Verification items for the finished model (mm, model axes). Face numbers are marked on the shaded views. A direction names the side the tool comes from. Round coordinates to 2 decimals unless told otherwise and drop trailing zeros. Write each loop counter-clockwise with the first axis right and the second up, starting at its lowest first coordinate (ties: lowest second). Pieces come first, ordered by that corner, then holes. Notation, with made-up numbers: (68.25, -22) - (94.25, -22) arc R12 ccw to (94.25, -3) - close; hole circle Ø8 at (72, 68). An arc over 180 degrees is marked (long way). Answer as a JSON object with one key per item and string values.
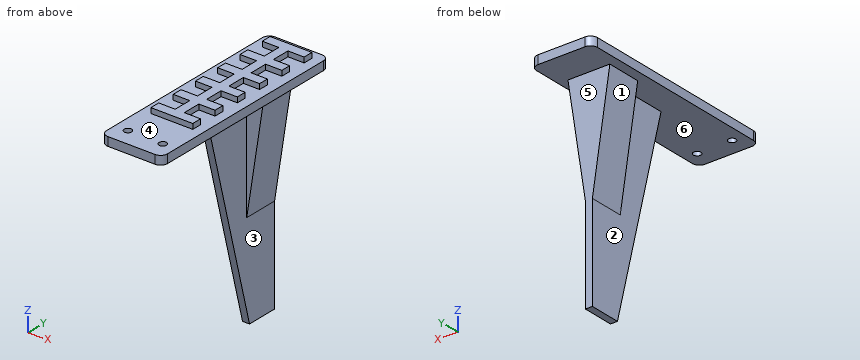
```python
from build123d import *

# Parameters (mm, degrees)
SKETCH1_W           = 15
SKETCH1_H           = 100
SKETCH1_W_2         = 35
SKETCH1_H_2         = 20
BOSS_EXTRUDE1_DEPTH = 5
SKETCH3_R           = 2.15
CUT_EXTRUDE1_DEPTH  = 6
BOSS_EXTRUDE3_DEPTH = 5
BOSS_EXTRUDE4_DEPTH = 2
BOSS_EXTRUDE5_DEPTH = 5
BOSS_EXTRUDE6_DEPTH = 20
FILLET3_R           = 4
BOSS_EXTRUDE7_DEPTH = 3


with BuildPart() as part:
    # Sketch1 → Boss-Extrude1 (new body)
    with BuildSketch(Plane.XY):
        with Locations((17.5, 50)):
            Rectangle(SKETCH1_W, SKETCH1_H)
        with Locations((17.5, -10)):
            Rectangle(SKETCH1_W_2, SKETCH1_H_2)
    extrude(amount=BOSS_EXTRUDE1_DEPTH)

    # Sketch3 → Cut-Extrude1 (cut, through all)
    with BuildSketch(Plane(origin=(0, 0, 0), x_dir=(-1, 0, 0), z_dir=(0, 0, -1))):
        with Locations((-27.5, -10)):
            Circle(SKETCH3_R)
        with Locations((-7.5, -10)):
            Circle(SKETCH3_R)
    extrude(amount=-CUT_EXTRUDE1_DEPTH, mode=Mode.SUBTRACT)

    # Sketch4 → Boss-Extrude3 (add)
    with BuildSketch(Plane(origin=(0, 0, 0), x_dir=(-1, 0, 0), z_dir=(0, 0, -1))):
        Polygon((-35, 0), (-25, 0), (-25, 62), align=None)
        Polygon((-10, 62), (0, 0), (-10, 0), align=None)
    extrude(amount=-BOSS_EXTRUDE3_DEPTH)

    # Sketch5 → Boss-Extrude4 (add, symmetric)
    with BuildSketch(Plane.ZY.offset(-17.5)):
        Polygon((0, 80.291537197), (0, 31), (-120, 62.291537197), (-120, 80.291537197), align=None)
    extrude(amount=BOSS_EXTRUDE4_DEPTH, both=True)

    # Sketch6 → Boss-Extrude5 (add)
    with BuildSketch(Plane.XY.offset(5)):
        Polygon((35, 100), (35, 0), (25, 62), (25, 100), align=None)
        Polygon((10, 100), (0, 100), (0, 0), (10, 62), align=None)
    extrude(amount=-BOSS_EXTRUDE5_DEPTH)

    # Sketch7 → Boss-Extrude6 (add)
    with BuildSketch(Plane(origin=(0, 80.291537197, 0), x_dir=(1, 0, 0), z_dir=(0, 1, 0))):
        Polygon((15.5, 65), (15.5, 0), (5.5, 0), align=None)
        Polygon((19.5, 0), (29.5, 0), (19.5, 65), align=None)
    extrude(amount=-BOSS_EXTRUDE6_DEPTH)

    # Fillet3
    fillet3_edges = [part.edges().sort_by_distance(p)[0] for p in [
        (35, -20, 2.5),
        (0, -20, 2.5),
        (35, 100, 2.5),
        (0, 100, 2.5),
    ]]
    fillet(fillet3_edges, radius=FILLET3_R)

    # Sketch8 → Boss-Extrude7 (add)
    with BuildSketch(Plane.XY.offset(5)):
        Polygon((14.979978143, 14.595461976), (5.5, 14.595461976), (5.5, 8.99207654), (29.5, 8.99207654), (29.5, 14.595461976), (20.184726016, 14.595461976), (20.184726016, 24.99207654), (29.5, 24.99207654), (29.5, 30.595461976), (20.184726016, 30.595461976), (20.184726016, 40.99207654), (29.5, 40.99207654), (29.5, 46.595461976), (20.184726016, 46.595461976), (20.184726016, 56.99207654), (29.5, 56.99207654), (29.5, 62.595461976), (20.184726016, 62.595461976), (20.184726016, 72.99207654), (29.5, 72.99207654), (29.5, 78.595461976), (20.184726016, 78.595461976), (20.184726016, 88.99207654), (29.5, 88.99207654), (29.5, 94.595461976), (5.5, 94.595461976), (5.5, 88.99207654), (14.979978143, 88.99207654), (14.979978143, 78.595461976), (5.5, 78.595461976), (5.5, 72.99207654), (14.979978143, 72.99207654), (14.979978143, 62.595461976), (5.5, 62.595461976), (5.5, 56.99207654), (14.979978143, 56.99207654), (14.979978143, 46.595461976), (5.5, 46.595461976), (5.5, 40.99207654), (14.979978143, 40.99207654), (14.979978143, 30.595461976), (5.5, 30.595461976), (5.5, 24.99207654), (14.979978143, 24.99207654), align=None)
    extrude(amount=BOSS_EXTRUDE7_DEPTH)


solid = part.part
```
1. Cross-section at B-B (y = -10). Record the boundary of the cut face in (x, z).
Completed:
{"outline": "(0, 0) - (5.35, 0) - (5.35, 5) - (0, 5) - close; (9.65, 0) - (25.35, 0) - (25.35, 5) - (9.65, 5) - close; (29.65, 0) - (35, 0) - (35, 5) - (29.65, 5) - close"}
2. Mould release check, pull along Y, two halves, no side actions. Record for the marked faces 4, 5 and 6: released by +Y, released by -Y, zero draft, split by the parting line, or undercut.
Completed:
{"face 4": "undercut", "face 5": "released by +Y", "face 6": "zero draft"}
3. Cross-section at A-A (y = 29). Record the boundary of the cut face in (x, z).
Completed:
{"outline": "(0, 0) - (35, 0) - (35, 5) - (29.5, 5) - (29.5, 8) - (5.5, 8) - (5.5, 5) - (0, 5) - close"}
4. Cross-section at D-D (y = 44.5). Record the boundary of the cut face in (x, z).
Completed:
{"outline": "(0, 0) - (15.5, 0) - (15.5, -51.77) - (19.5, -51.77) - (19.5, 0) - (35, 0) - (35, 5) - (29.5, 5) - (29.5, 8) - (5.5, 8) - (5.5, 5) - (0, 5) - close"}
5. Material ranges on probe 1 along Y at (x, z) = (7.5, 3.6); probe 2 along X at (y, z) = (60, -27); probe 3 along Z at (x, y) = (5, 54), recorded low to high. Write a range as from..to.
Completed:
{"probe 1": "y = -20..-12.15, -7.85..100", "probe 2": "x = 15.5..19.5", "probe 3": "z = 0..5"}
6. Go/stop test with flat-tipped pins: pin 1 (10 mm diameter, centred on x = 13, z = -93.5, fed in from +Y); pin 2 (11 mm diameter, centred on x = 9, z = -23, fed in from -Y); pin 3 (1.5 mm diameter, centred on y = 38, z = 6.5, fed in from +X); pin 4 (10 mm diameter, centred on y = 50.5, z = -96.5, fed in from +X). Record where each tip stops, or that it passes through.
Completed:
{"pin 1": "stops at y = 80.29", "pin 2": "stops at y = 60.29", "pin 3": "stops at x = 20.18", "pin 4": "passes through"}
7. Access from +Z, -Z, +X, -X, +Y, -Y to the whole of each face (thin tool, end or side, straight path). Record for the marked faces 1, 2 and 3.
Completed:
{"face 1": "-Z, -X, +Y, -Y", "face 2": "-Z, -X, -Y", "face 3": "-Z, +X, -Y"}
8. Cross-section at C-C (z = -39). Record the boundary of the cut face in (x, y).
Completed:
{"outline": "(11.5, 60.29) - (15.5, 60.29) - (15.5, 41.17) - (19.5, 41.17) - (19.5, 60.29) - (23.5, 60.29) - (23.5, 80.29) - (11.5, 80.29) - close"}
